```python
from build123d import *

# Parameters (mm, degrees)
CROQUIS1_W              = 150
CROQUIS1_H              = 28
CROQUIS1_R              = 11
SALIENTE_EXTRUIR1_DEPTH = 10
CROQUIS2_W              = 150
CROQUIS2_H              = 28
CROQUIS2_R              = 9.5
SALIENTE_EXTRUIR2_DEPTH = 2
CHAFL_N1_SIZE           = 2
REDONDEO1_R             = 14
CORTAR_EXTRUIR1_REACH   = 78.948
CROQUIS3_R              = 1.5


with BuildPart() as part:
    # Croquis1 → Saliente-Extruir1 (new body)
    with BuildSketch(Plane(origin=(0, 0, 0), x_dir=(0, 1, 0), z_dir=(0, 0, 1))):
        Rectangle(CROQUIS1_W, CROQUIS1_H)
        with Locations(Location((0, 0, 0), (0, 0, 270))):
            Circle(CROQUIS1_R, mode=Mode.SUBTRACT)
        with Locations(Location((60, 0, 0), (0, 0, 270))):
            Circle(CROQUIS1_R, mode=Mode.SUBTRACT)
        with Locations(Location((-60, 0, 0), (0, 0, 270))):
            Circle(CROQUIS1_R, mode=Mode.SUBTRACT)
    extrude(amount=SALIENTE_EXTRUIR1_DEPTH)

    # Croquis2 → Saliente-Extruir2 (add)
    with BuildSketch(Plane(origin=(0, 0, 0), x_dir=(0, 1, 0), z_dir=(0, 0, 1))):
        Rectangle(CROQUIS2_W, CROQUIS2_H)
        with Locations(Location((0, 0, 0), (0, 0, 270))):
            Circle(CROQUIS2_R, mode=Mode.SUBTRACT)
        with Locations(Location((60, 0, 0), (0, 0, 270))):
            Circle(CROQUIS2_R, mode=Mode.SUBTRACT)
        with Locations(Location((-60, 0, 0), (0, 0, 270))):
            Circle(CROQUIS2_R, mode=Mode.SUBTRACT)
    extrude(amount=SALIENTE_EXTRUIR2_DEPTH)

    # Chaflán1
    chafl_n1_edges = [part.edges().sort_by_distance(p)[0] for p in [
        (14, 0, 0),
    ]]
    chamfer(chafl_n1_edges, length=CHAFL_N1_SIZE)

    # Redondeo1
    redondeo1_edges = [part.edges().sort_by_distance(p)[0] for p in [
        (14, 75, 6),
        (-14, 75, 5),
        (14, -75, 6),
        (-14, -75, 5),
    ]]
    fillet(redondeo1_edges, radius=REDONDEO1_R - 0.0001)  # a hair under: the kernel refuses the full size

    # Croquis3 → Cortar-Extruir1 (cut, up to next)
    with BuildSketch(Plane.XY.offset(10), mode=Mode.PRIVATE) as cortar_extruir1_sk1:
        with Locations((-7, 30)):
            Circle(CROQUIS3_R)
    cortar_extruir1_tool1 = extrude(cortar_extruir1_sk1.sketch, amount=-CORTAR_EXTRUIR1_REACH, mode=Mode.PRIVATE) & part.part
    # Croquis3 → Cortar-Extruir1 (cut, up to next)
    with BuildSketch(Plane.XY.offset(10), mode=Mode.PRIVATE) as cortar_extruir1_sk2:
        with Locations(Location((7, 30, 0), (0, 0, 180))):
            Circle(CROQUIS3_R)
    cortar_extruir1_tool2 = extrude(cortar_extruir1_sk2.sketch, amount=-CORTAR_EXTRUIR1_REACH, mode=Mode.PRIVATE) & part.part
    # Croquis3 → Cortar-Extruir1 (cut, up to next)
    with BuildSketch(Plane.XY.offset(10), mode=Mode.PRIVATE) as cortar_extruir1_sk3:
        with Locations((7, -30)):
            Circle(CROQUIS3_R)
    cortar_extruir1_tool3 = extrude(cortar_extruir1_sk3.sketch, amount=-CORTAR_EXTRUIR1_REACH, mode=Mode.PRIVATE) & part.part
    # Croquis3 → Cortar-Extruir1 (cut, up to next)
    with BuildSketch(Plane.XY.offset(10), mode=Mode.PRIVATE) as cortar_extruir1_sk4:
        with Locations(Location((-7, -30, 0), (0, 0, 180))):
            Circle(CROQUIS3_R)
    cortar_extruir1_tool4 = extrude(cortar_extruir1_sk4.sketch, amount=-CORTAR_EXTRUIR1_REACH, mode=Mode.PRIVATE) & part.part
    add(cortar_extruir1_tool1.solids().sort_by_distance((-7, 30, 10))[0], mode=Mode.SUBTRACT)
    add(cortar_extruir1_tool2.solids().sort_by_distance((7, 30, 10))[0], mode=Mode.SUBTRACT)
    add(cortar_extruir1_tool3.solids().sort_by_distance((7, -30, 10))[0], mode=Mode.SUBTRACT)
    add(cortar_extruir1_tool4.solids().sort_by_distance((-7, -30, 10))[0], mode=Mode.SUBTRACT)


solid = part.part
```
Could you check a few things on this model? Use its own coordinates, in mm. A direction names the side the tool comes from. Round coordinates to 2 decimals unless told otherwise and drop trailing zeros. Loops run counter-clockwise (first coordinate to the right, second up) from the corner with the lowest first, then second, coordinate; pieces in that order, holes last. Notation, with made-up numbers: (11, 38) - (17, 38) arc R21 ccw to (17, 52) - close; hole circle Ø9 at (-35.5, 71.5). An arc over 180 degrees is marked (long way). Answer as CSV lines item,"result".
1. I want a section at A-A on y = 0. List the corners of the cut face in (x, z) for me, then the cut area to 3 significant figures.
Filled in:
outline,"(-14, 0) - (-9.5, 0) - (-9.5, 2) - (-11, 2) - (-11, 10) - (-14, 10) - close; (9.5, 0) - (12, 0) - (14, 2) - (14, 10) - (11, 10) - (11, 2) - (9.5, 2) - close"
area,"64.0 mm^2"
2. Please list where these lines run through material, in increasing order: line 1 along Y through (x, z) = (0, 6.75); line 2 along Y through (x, z) = (8.25, 8); line 3 along Y through (x, z) = (-9.75, 3.75). Write a range as [from, to].
Filled in:
line 1,"y = [-75, -71], [-49, -11], [11, 49], [71, 75]"
line 2,"y = [-72.31, -67.28], [-52.72, -30.83], [-29.17, -7.28], [7.28, 29.17], [30.83, 52.72], [67.28, 72.31]"
line 3,"y = [-71.05, -65.09], [-54.91, -5.09], [5.09, 54.91], [65.09, 71.05]"
3. For pin 1 Ø11.5 at (x, y) = (0, 0) entering from -Z; pin 2 Ø3 at (x, z) = (-10, 6.5) entering from -Y; pin 3 Ø6.5 at (x, y) = (-5, -64.5) entering from +Z, each with a flat end and sliding along its axis, tell me the tip position at first contact or that it passes through.
Filled in:
pin 1,"passes through"
pin 2,"stops at y = -72.12"
pin 3,"stops at z = 2"
4. On a 3-axis mill with a long thin cutter (end or side, diameter ignored), from which of +Z, -Z, +X, -X, +Y, -Y can I reach the whole of each face in a straight line? I mean faces 1 (the face through (0, -70, 2)), 2 (the face through (-1.24, 69.42, 0.99)). Say none if no direction works.
Filled in:
face 1,"+Z"
face 2,"+Z, -Z"
5. I want a section at D-D on x = 1.5. List the corners of the cut face in (y, z) for me.
Filled in:
outline,"(-74.92, 0) - (-69.38, 0) - (-69.38, 2) - (-70.9, 2) - (-70.9, 10) - (-74.92, 10) - close; (-50.62, 0) - (-9.38, 0) - (-9.38, 2) - (-10.9, 2) - (-10.9, 10) - (-49.1, 10) - (-49.1, 2) - (-50.62, 2) - close; (9.38, 0) - (50.62, 0) - (50.62, 2) - (49.1, 2) - (49.1, 10) - (10.9, 10) - (10.9, 2) - (9.38, 2) - close; (69.38, 0) - (74.92, 0) - (74.92, 10) - (70.9, 10) - (70.9, 2) - (69.38, 2) - close"
6. I want a section at C-C on y = -30. List the corners of the cut face in (x, z) for me.
Filled in:
outline,"(-14, 0) - (-8.5, 0) - (-8.5, 10) - (-14, 10) - close; (-5.5, 0) - (5.5, 0) - (5.5, 10) - (-5.5, 10) - close; (8.5, 0) - (12, 0) - (14, 2) - (14, 10) - (8.5, 10) - close"
7. We'd pull the mould along X, two halves only. Please class faces 3 (the face through (-2.059, -69.274, 0.986)), 4 (the face through (-14, -1, 5)), 5 (the face through (10, 70.8, 5.1)): +X half, -X half, draft (parallel to the pull), parting line (faces both ways), or undercut.
Filled in:
face 3,"undercut"
face 4,"-X half"
face 5,"+X half"
8. I want a section at B-B on z = 5. Count the separate pieces of the cut face and the enclosed holes in it, then the cut area to 3 significant figures.
Filled in:
separate pieces,"1"
enclosed holes,"7"
area,"2,860 mm^2"
